Build history of the part. All positions in model axes, mm. A direction names the side the tool comes from. Coordinates: 2 decimals unless noted, no trailing zeros. Loops run counter-clockwise (first coordinate to the right, second up) from the corner with the lowest first, then second, coordinate; pieces in that order, holes last.
Item 1: 3-axis set-ups, long thin cutter, end or side, ignore diameter. For faces 1 (the face through (44, 4, 17.2)), 2 (the face through (-12.4, 0, 23.1)), 3 (the face through (44, 4, 27.2)), 4 (the face through (-6.534, 0.507, -46.704)), 5 (the face through (-20.29, 3.958, -23.974)): which of +Z, -Z, +X, -X, +Y, -Y reach the whole face in a straight line?
Item 2: Mould opens along Z. For faces 6 (the face through (-40.29, 4.1, 25.52)), 7 (the face through (14.193, 4.042, -31.471)), 8 (the face through (-1.08, 4.04, -33.05)), 9 (the face through (20.51, 4.04, 27.98)) say: released by +Z, released by -Z, zero draft, split by the parting line, or undercut.
Item 3: Drill centre lines: line 1 along Z through (x, y) = (-10, 7.25); line 2 along Z through (x, y) = (8, 3.5); line 3 along Y through (x, z) = (50, 24). Where is each one in solid material? Low to high.
Item 4: Cut at A-A (x = 40). List the corners of the cut face in (y, z), and give its area (3 significant figures).
Item 5: Flat gauge pins, fed straight in: pin 1 (3.5 mm diameter, centred on x = 40, y = 4, fed in from +Z); pin 2 (4 mm diameter, centred on y = 1.5, z = 21.5, fed in from -X); pin 3 (1 mm diameter, centred on x = 22, y = 2, fed in from -Z); pin 4 (3 mm diameter, centred on x = -15, y = 6.5, fed in from +Z). Where does each tip first touch, or does it go through?
from build123d import *

# Parameters (mm, degrees)
BOSS_EXTRUDE1_DEPTH = 8
SKETCH2_R           = 2.25
CUT_EXTRUDE1_DEPTH  = 103.535212939
SKETCH4_R           = 25
SKETCH4_R_2         = 2.75
CUT_EXTRUDE2_DEPTH  = 90.231796233
FILLET1_R           = 5
FILLET2_R           = 100
FILLET3_R           = 3.5
SKETCH5_R           = 2.25
CUT_EXTRUDE3_DEPTH  = 94.342548859
SKETCH6_R           = 2.25
CUT_EXTRUDE4_DEPTH  = 87.844060995
CHAMFER1_SIZE       = 1


with BuildPart() as part:
    # Sketch1 → Boss-Extrude1 (new body)
    with BuildSketch(Plane(origin=(0, 0, 0), x_dir=(1, 0, 0), z_dir=(0, 1, 0))):
        with BuildLine():
            Line((60, -27.2), (60, -17.2))
            Line((60, -17.2), (26.27952308, -17.2))
            ThreePointArc((26.27952308, -17.2), (30.553109939, 7.277417565), (15.703927322, 27.2))
            Line((15.703927322, 27.2), (-6.444109017, 65.561524227))
            Line((-6.444109017, 65.561524227), (-15.104363055, 60.561524227))
            Line((-15.104363055, 60.561524227), (1.755875405, 31.358734587))
            ThreePointArc((1.755875405, 31.358734587), (-21.578983454, 22.821060589), (-31.407854644, 0))
            Line((-31.407854644, 0), (-53.555890983, -38.361524227))
            Line((-53.555890983, -38.361524227), (-44.895636945, -43.361524227))
            Line((-44.895636945, -43.361524227), (-28.035398485, -14.158734587))
            ThreePointArc((-28.035398485, -14.158734587), (-8.974126484, -30.098478154), (15.703927322, -27.2))
            Line((15.703927322, -27.2), (60, -27.2))
        make_face()
    extrude(amount=BOSS_EXTRUDE1_DEPTH)

    # Sketch2 → Cut-Extrude1 (cut, through all)
    with BuildSketch(Plane(origin=(0, 0, 17.2), x_dir=(-1, 0, 0), z_dir=(0, 0, -1))):
        with Locations((-50, 4)):
            Circle(SKETCH2_R)
        with Locations((-40, 4)):
            Circle(SKETCH2_R)
    extrude(amount=-CUT_EXTRUDE1_DEPTH, mode=Mode.SUBTRACT)

    # Sketch4 → Cut-Extrude2 (cut, through all)
    with BuildSketch(Plane(origin=(0, 8, 0), x_dir=(1, 0, 0), z_dir=(0, 1, 0))):
        with Locations(Location((0, 0, 0), (0, 0, 270))):
            Circle(SKETCH4_R)
        with Locations(Location((25, -22.2, 0), (0, 0, 270))):
            Circle(SKETCH4_R_2)
        with Locations(Location((-31.725763964, -10.550635095, 0), (0, 0, 270))):
            Circle(SKETCH4_R_2)
        with Locations(Location((6.725763964, 32.750635095, 0), (0, 0, 270))):
            Circle(SKETCH4_R_2)
    extrude(amount=-CUT_EXTRUDE2_DEPTH, mode=Mode.SUBTRACT)

    # Fillet1
    fillet1_edges = [part.edges().sort_by_distance(p)[0] for p in [
        (-6.444109017, 4, -65.561524227),
        (-15.104363055, 4, -60.561524227),
        (-53.555890983, 4, 38.361524227),
        (-44.895636945, 4, 43.361524227),
        (60, 4, 17.2),
        (60, 4, 27.2),
    ]]
    fillet(fillet1_edges, radius=FILLET1_R - 0.0001)  # a hair under: the kernel refuses the full size

    # Fillet2
    fillet2_edges = [part.edges().sort_by_distance(p)[0] for p in [
        (15.703927322, 4, 27.2),
        (-31.407854644, 4, 0),
        (15.703927322, 4, -27.2),
    ]]
    fillet(fillet2_edges, radius=FILLET2_R)

    # Fillet3
    fillet3_edges = [part.edges().sort_by_distance(p)[0] for p in [
        (26.27952308, 4, 17.2),
        (-28.035398485, 4, 14.158734587),
        (1.755875405, 4, -31.358734587),
    ]]
    fillet(fillet3_edges, radius=FILLET3_R)

    # Sketch5 → Cut-Extrude3 (cut, through all)
    with BuildSketch(Plane(origin=(-14.895636945, 0, -8.6), x_dir=(0.49999999999999967, 0, -0.8660254037844388), z_dir=(0.8660254037844388, 0, 0.49999999999999967))):
        with Locations((-50, 4)):
            Circle(SKETCH5_R)
        with Locations((-40, 4)):
            Circle(SKETCH5_R)
    extrude(amount=-CUT_EXTRUDE3_DEPTH, mode=Mode.SUBTRACT)

    # Sketch6 → Cut-Extrude4 (cut, through all)
    with BuildSketch(Plane(origin=(14.895636945, 0, -8.6), x_dir=(0.5000000000000007, 0, 0.8660254037844384), z_dir=(-0.8660254037844383, 0, 0.5000000000000006))):
        with Locations((-50, 4)):
            Circle(SKETCH6_R)
        with Locations((-40, 4)):
            Circle(SKETCH6_R)
    extrude(amount=-CUT_EXTRUDE4_DEPTH, mode=Mode.SUBTRACT)

    # Chamfer1
    chamfer1_edges = [part.edges().sort_by_distance(p)[0] for p in [
        (14.084814681, 0, -31.611912354),
        (14.084814681, 8, -31.611912354),
        (-34.419126501, 0, 3.608148855),
        (-34.419126501, 8, 3.608148855),
        (20.33431182, 0, 28.003763498),
        (20.33431182, 8, 28.003763498),
        (-20.487421356, 0, -23.805858513),
        (-20.487421356, 8, -23.805858513),
        (-10.372767553, 0, 29.645556608),
        (-10.372767553, 8, 29.645556608),
        (30.860188909, 0, -5.839698096),
        (30.860188909, 8, -5.839698096),
        (-1.058220823, 0, -33.090959821),
        (-1.058220823, 8, -33.090959821),
        (-28.128501429, 0, 17.461926027),
        (-28.128501429, 8, 17.461926027),
        (29.186722253, 0, 15.629033795),
        (29.186722253, 8, 15.629033795),
        (0, 0, -25),
        (0, 8, -25),
        (1.558956478, 0, -51.699808173),
        (43.553619041, 0, 17.2),
        (43.99386901, 0, 27.2),
        (-36.672446466, 0, 29.118540516),
        (-45.552825488, 0, 24.499808173),
        (-6.881172576, 0, -46.318540516),
        (58.535563195, 0, 25.735563195),
        (58.535563195, 0, 18.664436805),
        (-45.431658018, 0, 41.36106635),
        (-51.555433105, 0, 37.825503154),
        (-13.103905177, 0, -60.025503154),
        (-6.98013009, 0, -63.56106635),
        (1.558956478, 8, -51.699808173),
        (-6.881172576, 8, -46.318540516),
        (-45.552825488, 8, 24.499808173),
        (-36.672446466, 8, 29.118540516),
        (43.99386901, 8, 27.2),
        (43.553619041, 8, 17.2),
        (58.535563195, 8, 25.735563195),
        (58.535563195, 8, 18.664436805),
        (-45.431658018, 8, 41.36106635),
        (-51.555433105, 8, 37.825503154),
        (-13.103905177, 8, -60.025503154),
        (-6.98013009, 8, -63.56106635),
    ]]
    chamfer(chamfer1_edges, length=CHAMFER1_SIZE)


solid = part.part
Filled sheet:
1. face 1: -Z, +X, +Y, -Y
1. face 2: +Z, -Z, +X, -X, -Y
1. face 3: +Z, +X, +Y, -Y
1. face 4: -X, -Y
1. face 5: -X, +Y, -Y
2. face 6: undercut
2. face 7: released by -Z
2. face 8: undercut
2. face 9: released by +Z
3. line 1: z = -63.16 to -52.22, -29.51 to -23.19, 23.19 to 29.51
3. line 2: z = -40.58 to -35.19, -30.31 to -23.69, 23.69 to 30.37
3. line 3: y = 0 to 1.75, 6.25 to 8
4. outline: (0, 18.2) - (1, 17.2) - (1.75, 17.2) - (1.75, 27.2) - (1, 27.2) - (0, 26.2) - close; (6.25, 17.2) - (7, 17.2) - (8, 18.2) - (8, 26.2) - (7, 27.2) - (6.25, 27.2) - close
4. area: 33.0 mm2
5. pin 1: passes through
5. pin 2: stops at x = -44.98
5. pin 3: stops at z = -22.94
5. pin 4: stops at z = 28.36
